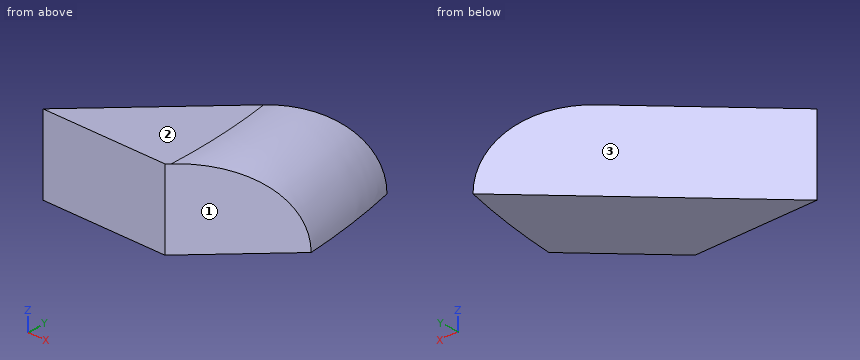
from build123d import *

# Parameters (mm, degrees)
F2_DEPTH = 25.4
F3_R     = 25.39999


# Not quite as in the source:
# - a fillet or chamfer is up to 0.001 mm smaller than in the source, because OpenCascade refuses the exact size


with BuildPart() as f2:
    # F1 (on face) → F2 (new body)
    with BuildSketch(Plane.XY):
        with BuildLine():
            Line((161.6446101792, 0), (202.0557627241, 0))
            Line((202.0557627241, 0), (227.2116647397, 25.1559020156))
            ThreePointArc((227.2116647397, 25.1559020156), (224.6556687953, 42.28227144), (220.8106438897, 59.1660337104))
            Line((220.8106438897, 59.1660337104), (161.6446101792, 0))
        make_face()
    extrude(amount=F2_DEPTH)

    # F3 (radius 25.4 in the source; OpenCascade refuses exactly that, so slightly less here)
    f3_edges = [f2.edges().sort_by_distance(p)[0] for p in [
        (224.655669, 42.282271, 25.4),
    ]]
    fillet(f3_edges, radius=F3_R)


solid = f2.part
CAD build for the part. Positions are in the model's coordinates, mm. Face numbers are marked on the shaded views. Round coordinates to 2 decimals unless told otherwise and drop trailing zeros. Order: outer loops, then holes, each group sorted by start corner. A loop starts at its lowest first (then second) coordinate and runs counter-clockwise, first axis right, second up. Notation, with made-up numbers: (44.5, -27.75) - (70.5, -27.75) arc R25 cw to (70.5, -13.75) - close; hole circle Ø1 at (42.5, 73.5). An arc over 180 degrees is marked (long way). Return JSON: item names as keys, results as strings.
(1) Pull direction Y, two halves, no side cores. Call the marked faces 1, 2 and 3: +Y half, -Y half, draft (parallel to the pull), parting line (faces both ways), or undercut.
Answer key:
{"face 1": "-Y half", "face 2": "draft", "face 3": "+Y half"}
(2) Cut at A-A (z = 20). Give the cut face in (x, y).
Answer key:
{"outline": "(161.64, 0) - (202.06, 0) - (218.26, 16.2) arc R218.86 ccw to (212.8, 51.15) - close"}
(3) Wall check: probe 1 along Z at (x, y) = (200.5, 35.5); probe 2 along X at (y, z) = (36.5, 19.5); probe 3 along Y at (x, z) = (204.5, 2.75). Give the ranges that are in metal, low to high. Write a range as from..to.
Answer key:
{"probe 1": "z = 0..25.4", "probe 2": "x = 198.14..216.42", "probe 3": "y = 2.44..42.86"}
(4) Cut at B-B (x = 169). Give the cut face in (y, z), then the cut area to 3 significant figures.
Answer key:
{"outline": "(0, 0) - (7.36, 0) - (7.36, 25.4) - (0, 25.4) - close", "area": "187 mm^2"}
(5) Pin check, flat tips, straight feed: pin 1 Ø3 at (x, z) = (204.5, 3) entering from -Y; pin 2 Ø3 at (x, z) = (197.5, 6.5) entering from +Y; pin 3 Ø2 at (x, z) = (204.5, 4.5) entering from -Y. Stop position of each tip, or through.
Answer key:
{"pin 1": "stops at y = 0.94", "pin 2": "stops at y = 37.36", "pin 3": "stops at y = 1.44"}
